Design review of the part built by this model. Coordinates are the model's own, in mm. Face numbers are marked on the shaded views. A direction names the side the tool comes from. Coordinates: 2 decimals unless noted, no trailing zeros. Write each loop counter-clockwise with the first axis right and the second up, starting at its lowest first coordinate (ties: lowest second). Pieces come first, ordered by that corner, then holes.
Q1. Take a section at A-A, the plane x = -47. Write out the cut boundary in (y, z).
Q2. The part is to be moulded in two halves that separate along X. For the marked faces 1, 2 and 3, say which applies: released by +X, released by -X, zero draft, split by the parting line, or undercut.
Q3. Take a section at C-C, the plane y = -20.5. Write out the cut boundary in (x, z).
Q4. For the marked faces 4 and 5, list the 3-axis set-ups (+Z, -Z, +X, -X, +Y, -Y) from which the entire face can be reached by the end or side of a thin tool; tool diameter is ignored.
Q5. Take a section at B-B, the plane x = 3.5. Write out the cut boundary in (y, z).
Q6. For pin 1 Ø2 at (x, z) = (-15.5, 2) entering from +Y, flat-tipped, find the tip position at first contact; note if it passes through.
Q7. Take a section at D-D, the plane x = -33. Write out the cut boundary in (y, z), plus the area to 3 significant figures.
Q8. For L1, parallel to X at y = 5, z = 3.65; L2, parallel to X at y = 11, z = 3.8; L3, parallel to Y at x = -29.5, z = 3.65, list the stretches that pass through material, from the lowest coordinate up.
Autodesk Inventor part; units mm, degrees
ref_plane "YZ Plane" through (0, 0, 0) normal (1, 0, 0) x (0, 1, 0)
ref_plane "XZ Plane" through (0, 0, 0) normal (0, 1, 0) x (-1, 0, 0)
ref_plane "XY Plane" through (0, 0, 0) normal (0, 0, 1) x (1, 0, 0)
sketch "Sketch1" plane through (0, 0, 0) normal (0, 0, 1) x (1, 0, 0)
  line L0 (-42.4511, 36.83) -> (-26.4283, 36.83)
  arc A0 (-24.6322, 36.0861) -> (-26.4283, 36.83) centre (-26.4283, 34.29) ccw
  line L1 (-24.6322, 36.0861) -> (-21.0157, 32.4696)
  arc A1 (-23.5785, 28.252) -> (-21.0157, 32.4696) centre (-22.8118, 30.6735) ccw
  line L2 (-23.5785, 28.252) -> (-42.8345, 34.3492)
  arc A2 (-42.4511, 36.83) -> (-42.8345, 34.3492) centre (-42.4511, 35.56) ccw
  line L3 (-42.8345, -8.9492) -> (-23.5785, -2.852)
  arc A3 (-21.0157, -7.0696) -> (-23.5785, -2.852) centre (-22.8118, -5.2735) ccw
  line L4 (-21.0157, -7.0696) -> (-24.6322, -10.6861)
  arc A4 (-26.4283, -11.43) -> (-24.6322, -10.6861) centre (-26.4283, -8.89) ccw
  line L5 (-26.4283, -11.43) -> (-42.4511, -11.43)
  arc A5 (-42.8345, -8.9492) -> (-42.4511, -11.43) centre (-42.4511, -10.16) ccw
  line L6 (-52.9416, -3.8174) -> (-52.9416, 29.2174)
  arc A6 (-48.8082, 32.2443) -> (-52.9416, 29.2174) centre (-49.7666, 29.2174) ccw
  line L7 (-48.8082, 32.2443) -> (-25.2598, 24.7879)
  arc A7 (-23.0433, 21.7611) -> (-25.2598, 24.7879) centre (-26.2183, 21.7611) ccw
  line L8 (-23.0433, 21.7611) -> (-23.0433, 3.6389)
  arc A8 (-25.2598, 0.6121) -> (-23.0433, 3.6389) centre (-26.2183, 3.6389) ccw
  line L9 (-25.2598, 0.6121) -> (-48.8082, -6.8443)
  arc A9 (-52.9416, -3.8174) -> (-48.8082, -6.8443) centre (-49.7666, -3.8174) ccw
  line L10 (-6.35, 22.8627) -> (-6.35, 2.5373)
  arc A10 (-7.3432, 0.2307) -> (-6.35, 2.5373) centre (-9.525, 2.5373) ccw
  line L11 (-7.3432, 0.2307) -> (-9.3482, -1.6658)
  arc A11 (-13.775, -1.6043) -> (-9.3482, -1.6658) centre (-11.53, 0.6408) ccw
  line L12 (-13.775, -1.6043) -> (-15.7633, 0.384)
  arc A12 (-16.6933, 2.629) -> (-15.7633, 0.384) centre (-13.5183, 2.629) ccw
  line L13 (-16.6933, 2.629) -> (-16.6933, 22.771)
  arc A13 (-15.7633, 25.016) -> (-16.6933, 22.771) centre (-13.5183, 22.771) ccw
  line L14 (-15.7633, 25.016) -> (-13.775, 27.0043)
  arc A14 (-9.3482, 27.0658) -> (-13.775, 27.0043) centre (-11.53, 24.7592) ccw
  line L15 (-9.3482, 27.0658) -> (-7.3432, 25.1693)
  arc A15 (-6.35, 22.8627) -> (-7.3432, 25.1693) centre (-9.525, 22.8627) ccw
  circle A16 centre (-55.8683, 24.7103) radius 1.27
  circle A17 centre (-55.8683, 0.7103) radius 1.27
  circle A18 centre (-19.8683, -11.2897) radius 1.27
  circle A19 centre (-19.8683, 12.7103) radius 1.27
  circle A20 centre (-19.8683, 36.7103) radius 1.27
  circle A21 centre (-19.8683, 24.7103) radius 1.27
  circle A22 centre (-19.8683, 0.7103) radius 1.27
  circle A23 centre (-55.8683, -11.2897) radius 1.27
  circle A24 centre (-55.8683, 12.7103) radius 1.27
  circle A25 centre (-55.8683, 36.7103) radius 1.27
  arc A26 (-54.2116, 40.64) -> (-59.2916, 35.56) centre (-54.2116, 35.56) ccw
  line L16 (-59.2916, -10.16) -> (-59.2916, 35.56)
  arc A27 (-59.2916, -10.16) -> (-54.2116, -15.24) centre (-54.2116, -10.16) ccw
  line L17 (-18.1336, -15.24) -> (-54.2116, -15.24)
  line L18 (0, 0) -> (0, 25.4) construction
  line L19 (-14.6427, 39.2505) -> (0, 25.4)
  arc A28 (-14.6427, 39.2505) -> (-18.1336, 40.64) centre (-18.1336, 35.56) ccw
  line L20 (-54.2116, 40.64) -> (-18.1336, 40.64)
  line L21 (0, 25.4) -> (10.5833, 15.3892)
  line L22 (10.5833, 15.3892) -> (10.5833, -42.7021)
  circle A29 centre (2.1167, 11.7435) radius 3.175
  line L23 (2.1167, 11.7435) -> (2.1167, -39.0565) construction
  circle A30 centre (2.1167, -39.0565) radius 3.175
  line L24 (-0.6484, -53.3263) -> (10.5833, -42.7021)
  line L25 (-18.1336, -15.24) -> (-0.6484, -53.3263)
  circle A31 centre (2.1167, -5.1898) radius 3.175
  circle A32 centre (2.1167, -22.1231) radius 3.175
  dimension "d0" = 8.4667
  dimension "d1" = 8.4667
  dimension "d2" = 8.4667
  dimension "d6" = 8.4667
  dimension "d7" = 6.35
  dimension "d10" = 50.8
  dimension "d11" = 8.4667
  dimension "d12" = 16.9333
  dimension "d13" = 16.9333
  dimension "d22" = 16.9333
extrude "Plate2" add sketch "Sketch1" along normal blind 5.08
fillet "Fillet1" radius 6.35 4 edges at (-18.1336, -15.24, 2.54) (-0.6484, -53.3263, 2.54) (10.5833, -42.7021, 2.54) (10.5833, 15.3892, 2.54)
sketch "Sketch2" plane through (0, 0, 5.08) normal (0, 0, 1) x (1, 0, 0)
  line L0 (-6.35, -4.0743) -> (-15.2168, -12.4614)
  line L1 (-15.2168, -12.4614) -> (-6.35, -31.7753)
  line L2 (-6.35, -31.7753) -> (-6.35, -4.0743)
  line L3 (-6.35, 22.8627) -> (-6.35, 2.5373)
  line L4 (-22.2055, -15.24) -> (-54.2116, -15.24)
  line L5 (-26.4283, -11.43) -> (-42.4511, -11.43)
  line L6 (-4.3455, -45.2733) -> (-16.4346, -18.9406)
  line L7 (-7.3432, 0.2307) -> (-9.3482, -1.6658)
  point P0 (0, 0)
  dimension "d15" = 3.81
  dimension "d16" = 3.81
  dimension "d17" = 3.81
extrude "Extrusion1" cut sketch "Sketch2" against normal blind 25.4
fillet "Fillet2" radius 1.778 2 edges at (-6.35, -31.7753, 2.54) (-6.35, -4.0743, 2.54)
fillet "Fillet3" radius 2.54 1 edges at (-15.2168, -12.4614, 2.54)
equation "\"d13\" = d12"
equation "\"d22\" = d12"
equation "\"d14\" = Thickness"
equation "\"BendRadius\" = Thickness"
equation "\"BendReliefWidth\" = Thickness"
equation "\"BendReliefDepth\" = 0.5 * Thickness"
equation "\"CornerReliefSize\" = 4 * Thickness"
equation "\"MinimumRemnant\" = 2 * Thickness"
equation "\"TransitionRadius\" = BendRadius"
equation "\"JacobiRadiusSize\" = BendRadius"
equation "\"GapSize\" = Thickness"
properties part number "UpperShoulderBracket"
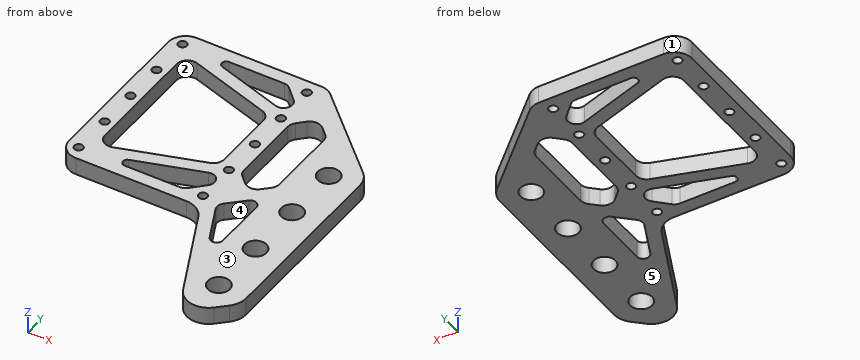
Responses:
1. outline: (-15.24, 0) - (-6.27, 0) - (-6.27, 5.08) - (-15.24, 5.08) - close; (31.67, 0) - (40.64, 0) - (40.64, 5.08) - (31.67, 5.08) - close
2. face 1: released by -X
2. face 2: undercut
2. face 3: zero draft
3. outline: (-15.72, 0) - (-11.53, 0) - (-11.53, 5.08) - (-15.72, 5.08) - close; (-6.35, 0) - (-0.61, 0) - (-0.61, 5.08) - (-6.35, 5.08) - close; (4.85, 0) - (10.58, 0) - (10.58, 5.08) - (4.85, 5.08) - close
4. face 4: +Z, -Z
4. face 5: -Z, +X, -X, +Y, -Y
5. outline: (-48.63, 0) - (-41.91, 0) - (-41.91, 5.08) - (-48.63, 5.08) - close; (-36.2, 0) - (-24.98, 0) - (-24.98, 5.08) - (-36.2, 5.08) - close; (-19.27, 0) - (-8.05, 0) - (-8.05, 5.08) - (-19.27, 5.08) - close; (-2.33, 0) - (8.89, 0) - (8.89, 5.08) - (-2.33, 5.08) - close; (14.6, 0) - (22.09, 0) - (22.09, 5.08) - (14.6, 5.08) - close
6. pin 1: stops at y = 40.37
7. outline: (-15.24, 0) - (-11.43, 0) - (-11.43, 5.08) - (-15.24, 5.08) - close; (-5.84, 0) - (-1.84, 0) - (-1.84, 5.08) - (-5.84, 5.08) - close; (27.24, 0) - (31.24, 0) - (31.24, 5.08) - (27.24, 5.08) - close; (36.83, 0) - (40.64, 0) - (40.64, 5.08) - (36.83, 5.08) - close
7. area: 79.3 mm2
8. L1: x = -59.29 to -52.94, -23.04 to -16.69, -6.35 to 10.58
8. L2: x = -59.29 to -52.94, -23.04 to -16.69, -6.35 to -0.97, 5.2 to 10.58
8. L3: y = -15.24 to -11.43, -4.73 to -0.73, 26.13 to 30.13, 36.83 to 40.64
